Part model, mm, in its own coordinate system. Face numbers are marked on the shaded views. Round coordinates to 2 decimals unless told otherwise and drop trailing zeros. Loops run counter-clockwise (first coordinate to the right, second up) from the corner with the lowest first, then second, coordinate; pieces in that order, holes last.
1) Band-saw the part on D-D, the plane x = 1.6. Write the cut outline in (y, z), then the cut area to 3 significant figures.
2) Band-saw the part on C-C, the plane y = 4. Write the cut outline in (x, z), then the cut area to 3 significant figures.
3) Drop flat-ended pins along their axis: P1, Ø2, axis at x = 1.5, z = -4, coming from the +Y side; P2, Ø3, axis at x = -2, y = 3.5, coming from the -Z side. Give the stop position or say it passes through.
4) Mould opens along X. For the marked faces 1, 2, 3 and 4 say: +X half, -X half, draft (parallel to the pull), parting line (faces both ways), or undercut.
5) Band-saw the part on B-B, the plane z = 2.6. Write the cut outline in (x, y), then the cut area to 3 significant figures.
6) Band-saw the part on A-A, the plane x = 0. Write the cut outline in (y, z).
7) Probe line 1 (X direction, y = 4, z = -2.9); line 2 (Z direction, x = 2.1, y = 2); line 3 (Z direction, x = -1.15, y = 6.5). List the from-to ranges inside material, lowest first.
from build123d import *

# Parameters (mm, degrees)
SKETCH4_W           = 6
SKETCH4_H           = 12
BOSS_EXTRUDE2_DEPTH = 7
SKETCH5_R           = 2.35
SKETCH5_R_2         = 2.5
CUT_EXTRUDE2_DEPTH  = 10.695359715
CUT_EXTRUDE3_DEPTH  = 10.695359715


with BuildPart() as part:
    # Sketch4 → Boss-Extrude2 (new body)
    with BuildSketch(Plane(origin=(0, 0, 0), x_dir=(1, 0, 0), z_dir=(0, 1, 0))):
        Rectangle(SKETCH4_W, SKETCH4_H)
    extrude(amount=BOSS_EXTRUDE2_DEPTH)

    # Sketch5 → Cut-Extrude2 (cut, through all)
    with BuildSketch(Plane(origin=(0, 7, 0), x_dir=(1, 0, 0), z_dir=(0, 1, 0))):
        with Locations(Location((0, -2.6, 0), (0, 0, 270))):
            Circle(SKETCH5_R)
        with Locations(Location((0, 2.9, 0), (0, 0, 270))):
            Circle(SKETCH5_R_2)
    extrude(amount=-CUT_EXTRUDE2_DEPTH, mode=Mode.SUBTRACT)

    # Sketch7 → Cut-Extrude3 (cut, through all)
    with BuildSketch(Plane(origin=(0, 7, 0), x_dir=(1, 0, 0), z_dir=(0, 1, 0))):
        with BuildLine():
            Line((-3, 2.9), (-3, 6))
            Line((-3, 6), (3, 6))
            Line((3, 6), (3, 2.9))
            ThreePointArc((3, 2.9), (0, 5.9), (-3, 2.9))
        make_face()
    extrude(amount=-CUT_EXTRUDE3_DEPTH, mode=Mode.SUBTRACT)


solid = part.part
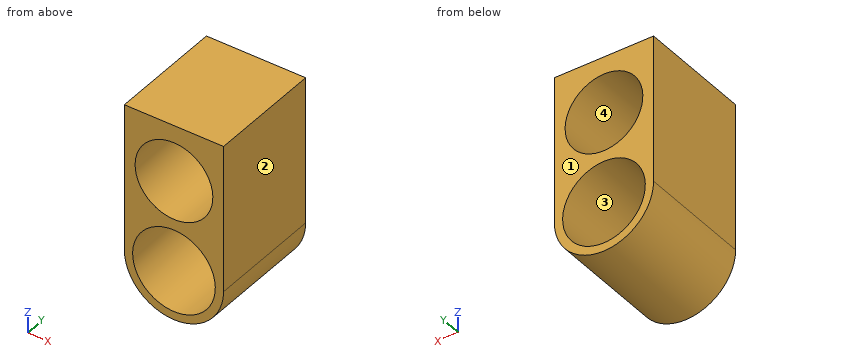
Reported:
1. outline: (0, -5.44) - (7, -5.44) - (7, -4.82) - (0, -4.82) - close; (0, -0.98) - (7, -0.98) - (7, 0.88) - (0, 0.88) - close; (0, 4.32) - (7, 4.32) - (7, 6) - (0, 6) - close
1. area: 29.1 mm2
2. outline: (-3, -2.9) arc R3 ccw to (3, -2.9) - (3, 6) - (-3, 6) - close; hole circle Ø5 at (0, -2.9); hole circle Ø4.7 at (0, 2.6)
2. area: 30.6 mm2
3. P1: stops at y = 7
3. P2: stops at z = -5.86
4. face 1: draft
4. face 2: +X half
4. face 3: undercut
4. face 4: undercut
5. outline: (-3, 0) - (-2.35, 0) - (-2.35, 7) - (-3, 7) - close; (2.35, 0) - (3, 0) - (3, 7) - (2.35, 7) - close
5. area: 9.10 mm2
6. outline: (0, -5.9) - (7, -5.9) - (7, -5.4) - (0, -5.4) - close; (0, -0.4) - (7, -0.4) - (7, 0.25) - (0, 0.25) - close; (0, 4.95) - (7, 4.95) - (7, 6) - (0, 6) - close
7. line 1: x = -3 to -2.5, 2.5 to 3
7. line 2: z = -5.04 to -4.26, -1.54 to 1.55, 3.65 to 6
7. line 3: z = -5.67 to -5.12, -0.68 to 0.55, 4.65 to 6
